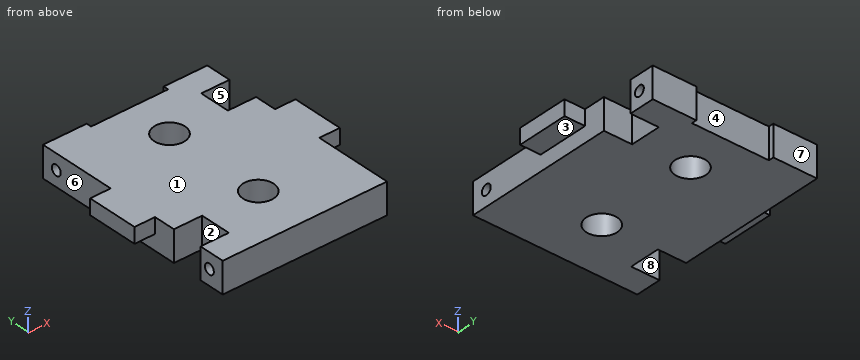
```python
from build123d import *

# Parameters (mm, degrees)
SKETCH_1_R          = 3
EXTRUDE_1_DEPTH     = 3
EXTRUDE_START       = -6
SKETCH_2_R          = 3
EXTRUDE_2_DEPTH     = 6
SKETCH_3_R          = 1
CUT_EXTRUDE_1_DEPTH = 55.270157545
SKETCH_6_W          = 15
SKETCH_6_H          = 1
CUT_EXTRUDE_5_DEPTH = 10


with BuildPart() as part:
    # 草图1 → 凸台-拉伸1 (new body)
    with BuildSketch(Plane.XY):
        Polygon((0, 0), (0, -15.25), (-4, -15.25), (-4, -25.25), (0, -25.25), (0, -29.5), (5.5, -29.5), (5.5, -35.5), (0, -35.5), (0, -40.5), (32, -40.5), (32, -25.25), (36, -25.25), (36, -15.25), (32, -15.25), (32, -11), (26.5, -11), (26.5, -5), (32, -5), (32, 0), align=None)
        with Locations((16, -10)):
            Circle(SKETCH_1_R, mode=Mode.SUBTRACT)
        with Locations((16, -30)):
            Circle(SKETCH_1_R, mode=Mode.SUBTRACT)
    extrude(amount=EXTRUDE_1_DEPTH)

    # 草图2 → 凸台-拉伸2 (add)
    with BuildSketch(Plane.XY.offset(3).offset(EXTRUDE_START)):
        Polygon((0, 0), (0, -29.5), (5.5, -29.5), (5.5, -35.5), (0, -35.5), (0, -40.5), (32, -40.5), (32, -11), (26.5, -11), (26.5, -5), (32, -5), (32, 0), align=None)
        with Locations((16, -10)):
            Circle(SKETCH_2_R, mode=Mode.SUBTRACT)
        with Locations((16, -30)):
            Circle(SKETCH_2_R, mode=Mode.SUBTRACT)
    extrude(amount=EXTRUDE_2_DEPTH)

    # 草图3 → 切除-拉伸1 (cut, through all)
    with BuildSketch(Plane(origin=(32, 0, 0), x_dir=(0, 0, -1), z_dir=(1, 0, 0))):
        with Locations((0, -3)):
            Circle(SKETCH_3_R)
        with Locations((0, -37.5)):
            Circle(SKETCH_3_R)
    extrude(amount=-CUT_EXTRUDE_1_DEPTH, mode=Mode.SUBTRACT)

    # 草图6 → 切除-拉伸5 (cut)
    with BuildSketch(Plane.XY.offset(3)):
        with Locations((16, -0.5)):
            Rectangle(SKETCH_6_W, SKETCH_6_H)
    extrude(amount=-CUT_EXTRUDE_5_DEPTH, mode=Mode.SUBTRACT)


solid = part.part
```
CAD build for the part. Positions are in the model's coordinates, mm. Face numbers are marked on the shaded views. A direction names the side the tool comes from. Coordinates: 2 decimals unless noted, no trailing zeros. Write each loop counter-clockwise with the first axis right and the second up, starting at its lowest first coordinate (ties: lowest second). Pieces come first, ordered by that corner, then holes. Notation, with made-up numbers: (70, 40) -> (88, 40) arc R11 cw to (88, 48) -> close; hole circle Ø5 at (9, 83.25). An arc over 180 degrees is marked (long way). Return JSON: item names as keys, results as strings. Group by question number.
Q1. Cut at D-D, the plane y = -21. Give the cut face in (x, z), then the cut area to 3 significant figures.
Q2. Drill centre lines: line 1 (Y direction, x = 16, z = -1.9); line 2 (Y direction, x = 11, z = -0.2); line 3 (Y direction, x = 18, z = 0). Where is each one in solid material? Low to high.
Q3. Cut at A-A, the plane x = 27.5. Give the cut face in (y, z).
Q4. Cut at B-B, the plane y = -3. Give the cut face in (x, z), then the cut area to 3 significant figures.
Q5. Pull direction Y, two halves, no side cores. Call the marked faces 6, 7 and 8: released by +Y, released by -Y, zero draft, split by the parting line, or undercut.
Q6. Flat gauge pins, fed straight in: pin 1 (2.5 mm diameter, centred on y = -3, z = 0, fed in from -X); pin 2 (2 mm diameter, centred on y = -32.5, z = 1.5, fed in from +X); pin 3 (5.5 mm diameter, centred on x = 16, y = -10, fed in from +Z); pin 4 (4.5 mm diameter, centred on x = 34.5, y = -19, fed in from -Z). Where does each tip first touch, or does it go through?
Q7. Which spindle directions (+Z, -Z, +X, -X, +Y, -Y) get a long thin tool onto all of the face, cutting with end or side? Do the marked faces 1, 2, 3, 4 and 5. Say none if no direction does.
Q8. Cut at C-C, the plane z = -1.9. Give the cut face in (x, y), then the cut area to 3 significant figures.
Returned:
{
 "1": {"outline": "(-4, 0) -> (0, 0) -> (0, -3) -> (32, -3) -> (32, 0) -> (36, 0) -> (36, 3) -> (-4, 3) -> close", "area": "216 mm2"},
 "2": {"line 1": "y = -40.5 to -33, -27 to -13, -7 to -1", "line 2": "y = -40.5 to -38.48, -36.52 to -3.98, -2.02 to -1", "line 3": "y = -40.5 to -38.5, -36.5 to -32.24, -27.76 to -12.24, -7.76 to -4, -2 to -1"},
 "3": {"outline": "(-40.5, -3) -> (-11, -3) -> (-11, 3) -> (-40.5, 3) -> close; (-5, -3) -> (0, -3) -> (0, 3) -> (-5, 3) -> close; hole circle Ø2 at (-37.5, 0); hole circle Ø2 at (-3, 0)"},
 "4": {"outline": "(0, -3) -> (32, -3) -> (32, -1) -> (0, -1) -> close; (0, 1) -> (32, 1) -> (32, 3) -> (0, 3) -> close", "area": "128 mm2"},
 "5": {"face 6": "zero draft", "face 7": "released by +Y", "face 8": "undercut"},
 "6": {"pin 1": "stops at x = 0", "pin 2": "stops at x = 32", "pin 3": "passes through", "pin 4": "stops at z = 0"},
 "7": {"face 1": "+Z, +X, -X, +Y, -Y", "face 2": "+Z, -Z, -X", "face 3": "-Z, +X, +Y, -Y", "face 4": "+Z, -Z, +Y", "face 5": "+Z, -Z, +X"},
 "8": {"outline": "(0, -40.5) -> (32, -40.5) -> (32, -11) -> (26.5, -11) -> (26.5, -5) -> (32, -5) -> (32, 0) -> (23.5, 0) -> (23.5, -1) -> (8.5, -1) -> (8.5, 0) -> (0, 0) -> (0, -29.5) -> (5.5, -29.5) -> (5.5, -35.5) -> (0, -35.5) -> close; hole circle Ø6 at (16, -30); hole circle Ø6 at (16, -10)", "area": "1,160 mm2"}
}
